Read the model definition and answer for the solid it produces. Units are mm, in the model's axes. A direction names the side the tool comes from. Give positions to 0.01 mm unless a question says otherwise; leave off trailing zeros. Loops run counter-clockwise (first coordinate to the right, second up) from the corner with the lowest first, then second, coordinate; pieces in that order, holes last. Notation, with made-up numbers: M -40,40 L 8,40 A7 cw 8,49 Z; hole C 53.25,-11 d3. An arc over 180 degrees is marked long. Return JSON: item names as keys, results as strings. Group by question number.
Autodesk Inventor part; units mm, degrees
ref_plane "YZ Plane" through (0, 0, 0) normal (1, 0, 0) x (0, 1, 0)
ref_plane "XZ Plane" through (0, 0, 0) normal (0, 1, 0) x (-1, 0, 0)
ref_plane "XY Plane" through (0, 0, 0) normal (0, 0, 1) x (1, 0, 0)
sketch "Sketch1" plane through (0, 0, 0) normal (0, 1, 0) x (-1, 0, 0)
  arc A0 (-8.6603, -5) -> (-8.6603, 5) centre (0, 0) ccw
  line L0 (-8.6603, -5) -> (-16, -9.2376)
  line L1 (-8.6603, 5) -> (-16, 9.2376)
  line L2 (0, 0) -> (23, 0)
  line L3 (23, 0) -> (23, -24)
  line L4 (23, 0) -> (23, 24)
  line L5 (23, -24) -> (-16, -24)
  line L6 (-16, -24) -> (-16, -9.2376)
  line L7 (23, 24) -> (-16, 24)
  line L8 (-16, 24) -> (-16, 9.2376)
  dimension "d0" = 20
  dimension "d2" = 23
  dimension "d3" = 24
  dimension "d4" = 24
  dimension "d5" = 39
extrude "Extrusion1" add sketch "Sketch1" along normal blind 50
sketch "Sketch2" plane through (-23, 0, -24) normal (-1, 0, 0) x (0, 0, 1)
  line L0 (48, 0) -> (48, 50)
  line L1 (14.7624, 0) -> (0, 0)
  line L2 (48, 0) -> (33.2376, 0)
  line L3 (14.7624, 50) -> (0, 50)
  circle A0 centre (6.5, 42.5) radius 3
  circle A1 centre (6.5, 7.5) radius 3
  circle A2 centre (41.5, 7.5) radius 3
  circle A3 centre (41.5, 42.5) radius 3
  point P0 (24, 0)
  point P1 (24, 25)
  dimension "d10" = 6
  dimension "d11" = 6
  dimension "d12" = 6
  dimension "d13" = 6
extrude "Extrusion2" cut sketch "Sketch2" against normal blind 12
properties part number "Rodamiento lineal"
1. For faces 4 (the flat face through (12.3, 24.6, -7.1)), 5 (the flat face through (-11, 43, 17)), 6 (the cylindrical face through (-10, 25, 0)), determine the directions among +Z, -Z, +X, -X, +Y, -Y from which every point of the face is accessible in a straight line to the end or side of a thin tool.
2. Find section D-D (x = -14). Write down the section's boundary in (y, z).
3. Flat-ended cylindrical pins translate along their axes: P1, Ø8, axis at y = 7.5, z = 17.5, coming from the -X side; P2, Ø3, axis at y = 6.5, z = -18.5, coming from the -X side. Find the tip coordinate at first contact, or state that the pin passes through.
4. Find section A-A (x = 0). Write down the section's boundary in (y, z).
5. The mould has two halves that part along Y. Classify faces 1 (the flat face through (-12, 50, 0)), 2 (the flat face through (-11, 8, -18)), 3 (the flat face through (12.3, 24.6, 7.1)): +Y half, -Y half, draft (parallel to the pull), parting line (faces both ways), or undercut.
6. Straight lines are drawn through the part: line 1 along Y through (x, z) = (-15.25, -17.5); line 2 along Z through (x, y) = (-18, 7); line 3 along Z through (x, y) = (3, 29.5). For each, find the intervals that lie inside material, in ascending order.
7. Find section B-B (y = 33). Write down the section's boundary in (x, z).
8. Find section C-C (z = -17.5). Write down the section's boundary in (x, y).
Result:
{
 "1": {"face 4": "+X, +Y, -Y", "face 5": "-X", "face 6": "+Y, -Y"},
 "2": {"outline": "M 0,-24 L 50,-24 L 50,24 L 0,24 Z; hole C 7.5,-17.5 d6; hole C 7.5,17.5 d6; hole C 42.5,-17.5 d6; hole C 42.5,17.5 d6"},
 "3": {"P1": "stops at x = -23", "P2": "stops at x = -11"},
 "4": {"outline": "M 0,-24 L 50,-24 L 50,-10 L 0,-10 Z; M 0,10 L 50,10 L 50,24 L 0,24 Z"},
 "5": {"face 1": "+Y half", "face 2": "undercut", "face 3": "draft"},
 "6": {"line 1": "y = 0 to 4.5, 10.5 to 39.5, 45.5 to 50", "line 2": "z = -24 to -20.46, -14.54 to 14.54, 20.46 to 24", "line 3": "z = -24 to -9.54, 9.54 to 24"},
 "7": {"outline": "M -23,-24 L 16,-24 L 16,-9.24 L 8.66,-5 A10 cw long 8.66,5 L 16,9.24 L 16,24 L -23,24 Z"},
 "8": {"outline": "M -23,0 L 16,0 L 16,50 L -23,50 L -23,45.5 L -11,45.5 L -11,39.5 L -23,39.5 L -23,10.5 L -11,10.5 L -11,4.5 L -23,4.5 Z"}
}
